Work out the finished part from the listing and answer in its coordinate system (mm). Face numbers are marked on the shaded views. A direction names the side the tool comes from. Coordinates: 2 decimals unless noted, no trailing zeros. Loops run counter-clockwise (first coordinate to the right, second up) from the corner with the lowest first, then second, coordinate; pieces in that order, holes last. Notation, with made-up numbers: (-8, 63.25) -> (32, 63.25) arc R31 ccw to (32, 87.25) -> close; hole circle Ø6 at (-21, -32.5). An arc over 180 degrees is marked (long way). One line per question, with ' | ' between items.
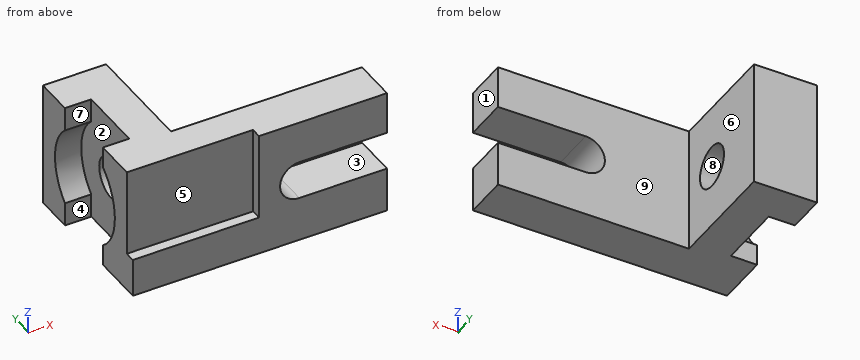
```python
from build123d import *

# Parameters (mm, degrees)
SKETCH1_W           = 145
SKETCH1_H           = 72
BOSS_EXTRUDE1_DEPTH = 25
SKETCH2_W           = 72
SKETCH2_H           = 6
CUT_EXTRUDE1_DEPTH  = 50
CUT_EXTRUDE2_DEPTH  = 50
SKETCH4_W           = 36
SKETCH4_H           = 65
BOSS_EXTRUDE2_DEPTH = 72
SKETCH5_R           = 30
CUT_EXTRUDE3_DEPTH  = 15
SKETCH6_W           = 15
SKETCH6_H           = 38
CUT_EXTRUDE4_DEPTH  = 137.162586638
SKETCH7_R           = 12
CUT_EXTRUDE5_DEPTH  = 163.160414405


with BuildPart() as part:
    # Sketch1 → Boss-Extrude1 (new body)
    with BuildSketch(Plane(origin=(0, 0, 0), x_dir=(1, 0, 0), z_dir=(0, 1, 0))):
        Rectangle(SKETCH1_W, SKETCH1_H)
    extrude(amount=BOSS_EXTRUDE1_DEPTH)

    # Sketch2 → Cut-Extrude1 (cut)
    with BuildSketch(Plane.XY.offset(36)):
        with Locations((-36.5, 3)):
            Rectangle(SKETCH2_W, SKETCH2_H)
    extrude(amount=-CUT_EXTRUDE1_DEPTH, mode=Mode.SUBTRACT)

    # Sketch3 → Cut-Extrude2 (cut)
    with BuildSketch(Plane(origin=(0, 25, 0), x_dir=(1, 0, 0), z_dir=(0, 1, 0))):
        with BuildLine():
            Line((22.5, 10.292135336), (72.5, 10.292135336))
            Line((72.5, 10.292135336), (72.5, -11.707864664))
            Line((72.5, -11.707864664), (22.5, -11.707864664))
            ThreePointArc((22.5, -11.707864664), (11.5, -0.707864664), (22.5, 10.292135336))
        make_face()
    extrude(amount=-CUT_EXTRUDE2_DEPTH, mode=Mode.SUBTRACT)

    # Sketch4 → Boss-Extrude2 (add)
    with BuildSketch(Plane.XY.offset(36)):
        with Locations((-54.5, 57.5)):
            Rectangle(SKETCH4_W, SKETCH4_H)
    extrude(amount=-BOSS_EXTRUDE2_DEPTH)

    # Sketch5 → Cut-Extrude3 (cut)
    with BuildSketch(Plane.ZY.offset(72.5)):
        with Locations((0, 48)):
            Circle(SKETCH5_R)
    extrude(amount=-CUT_EXTRUDE3_DEPTH, mode=Mode.SUBTRACT)

    # Sketch6 → Cut-Extrude4 (cut, through all)
    with BuildSketch(Plane.XY.offset(36)):
        with Locations((-65, 49)):
            Rectangle(SKETCH6_W, SKETCH6_H)
    extrude(amount=-CUT_EXTRUDE4_DEPTH, mode=Mode.SUBTRACT)

    # Sketch7 → Cut-Extrude5 (cut, through all)
    with BuildSketch(Plane.ZY.offset(57.5)):
        with Locations((0, 48)):
            Circle(SKETCH7_R)
    extrude(amount=-CUT_EXTRUDE5_DEPTH, mode=Mode.SUBTRACT)


solid = part.part
```
1) Find section C-C (x = -48.5). Write down the section's boundary in (y, z), plus the area to 3 significant figures.
Check values:
outline: (0, -36) -> (90, -36) -> (90, 36) -> (6, 36) -> (6, -14) -> (0, -14) -> close; hole circle Ø24 at (48, 0) | area: 5,730 mm^2
2) Find the intervals of material crossed by line 1 along Y through (x, z) = (-52, 0); line 2 along X through (y, z) = (25.5, 6); line 3 along Y through (x, z) = (-17, 2), in increasing order.
Check values:
line 1: y = 6 to 36, 60 to 90 | line 2: x = -57.5 to -36.5 | line 3: y = 6 to 25
3) The mould has two halves that part along Y. Classify the marked faces 6, 7, 8 and 9: released by +Y, released by -Y, zero draft, split by the parting line, or undercut.
Check values:
face 6: zero draft | face 7: undercut | face 8: undercut | face 9: released by +Y
4) Find section A-A (x = 29). Write down the section's boundary in (y, z), plus the area to 3 significant figures.
Check values:
outline: (0, -36) -> (25, -36) -> (25, -10.29) -> (0, -10.29) -> close; (0, 11.71) -> (25, 11.71) -> (25, 36) -> (0, 36) -> close | area: 1,250 mm^2
5) Find section D-D (z = 0). Write down the section's boundary in (x, y).
Check values:
outline: (-72.5, 6) -> (-0.5, 6) -> (-0.5, 0) -> (11.52, 0) -> (11.52, 25) -> (-36.5, 25) -> (-36.5, 36) -> (-57.5, 36) -> (-57.5, 18) -> (-72.5, 18) -> close; (-72.5, 78) -> (-57.5, 78) -> (-57.5, 60) -> (-36.5, 60) -> (-36.5, 90) -> (-72.5, 90) -> close
6) Find section B-B (y = 48). Write down the section's boundary in (x, z), plus the area to 3 significant figures.
Check values:
outline: (-57.5, -36) -> (-36.5, -36) -> (-36.5, -12) -> (-57.5, -12) -> close; (-57.5, 12) -> (-36.5, 12) -> (-36.5, 36) -> (-57.5, 36) -> close | area: 1,010 mm^2
7) For the marked faces 1, 2, 3, 4 and 5, determine the directions among +Z, -Z, +X, -X, +Y, -Y from which every point of the face is accessible in a straight line to the end or side of a thin tool.
Check values:
face 1: +Z, -Z, +X, +Y, -Y | face 2: -X | face 3: +X, +Y, -Y | face 4: +Z, -Z, -X | face 5: +Z, -X, -Y
8) Flat-ended cylindrical pins translate along their axes: pin 1 (7 mm diameter, centred on x = -66.5, z = 31, fed in from -Y); pin 2 (15 mm diameter, centred on x = -61.5, z = -31, fed in from -Y); pin 3 (8 mm diameter, centred on y = 45, z = -9.5, fed in from -X); pin 4 (1.8 mm diameter, centred on y = 3, z = 13.5, fed in from -X). Find the tip coordinate at first contact, or state that the pin passes through.
Check values:
pin 1: stops at y = 6 | pin 2: stops at y = 0 | pin 3: stops at x = -57.5 | pin 4: stops at x = -0.5
